The model under review builds one solid part; all positions refer to its coordinate system, in mm. Round coordinates to 2 decimals unless told otherwise and drop trailing zeros. Write each loop counter-clockwise with the first axis right and the second up, starting at its lowest first coordinate (ties: lowest second). Pieces come first, ordered by that corner, then holes.
Item 1: To check wall thickness, follow L1, parallel to Y at x = 187.5, z = 6; L2, parallel to Y at x = 100, z = 3; L3, parallel to Y at x = 35, z = 6.25. State the ranges of each line that lie inside material, in increasing order.
Item 2: Add section D-D (y = 137.3). Give the boundary of the cut face in (x, z).
Item 3: Add section A-A (y = 29). Give the boundary of the cut face in (x, z), plus the area to 3 significant figures.
Item 4: Clearance check with a flat-ended pin moving along its axis: pin 1 Ø4 at (x, z) = (15, 4) entering from -Y. State where the tip first meets the part, or that it passes through.
Item 5: Add section B-B (x = 100). Give the boundary of the cut face in (y, z).
Item 6: Add section C-C (x = 35). Give the boundary of the cut face in (y, z).
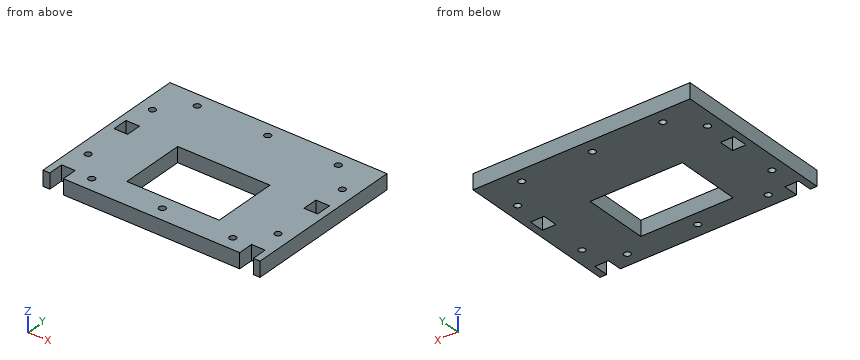
```python
from build123d import *

# Parameters (mm, degrees)
SKETCH1_W                = 200
SKETCH1_H                = 150
BOSS_EXTRUDE1_DEPTH      = 14
SKETCH2_W                = 12.5
SKETCH2_H                = 14
CUT_EXTRUDE1_DEPTH       = 14
F_6_0_6_DIAMETER_HOLE1_D = 6
SKETCH6_W                = 85
SKETCH6_H                = 60
CUT_EXTRUDE2_DEPTH       = 15


with BuildPart() as part:
    # Sketch1 → Boss-Extrude1 (new body)
    with BuildSketch(Plane.XY):
        with Locations((100, 75)):
            Rectangle(SKETCH1_W, SKETCH1_H)
    extrude(amount=BOSS_EXTRUDE1_DEPTH)

    # Sketch2 → Cut-Extrude1 (cut)
    with BuildSketch(Plane(origin=(0, 0, 0), x_dir=(-1, 0, 0), z_dir=(0, 0, -1))):
        with Locations((-12.5, 7)):
            Rectangle(SKETCH2_W, SKETCH2_H)
        with Locations((-187.5, 7)):
            Rectangle(SKETCH2_W, SKETCH2_H)
        with Locations((-12.5, 83)):
            Rectangle(SKETCH2_W, SKETCH2_H)
        with Locations((-187.5, 83)):
            Rectangle(SKETCH2_W, SKETCH2_H)
    extrude(amount=-CUT_EXTRUDE1_DEPTH, mode=Mode.SUBTRACT)

    # Ø6.0 (6) Diameter Hole1 (through all)
    with Locations(Plane.XY.offset(14)):
        with Locations((12.5, 113.265728709), (187.5, 113.265728709), (187.5, 37.265728709), (12.5, 37.265728709), (35, 137.3), (100, 137.3), (165, 137.3), (165, 12.7), (100, 12.7), (35, 12.7)):
            Hole(F_6_0_6_DIAMETER_HOLE1_D / 2)

    # Sketch6 → Cut-Extrude2 (cut, through all)
    with BuildSketch(Plane.XY.offset(14)):
        with Locations((100, 55.4)):
            Rectangle(SKETCH6_W, SKETCH6_H)
    extrude(amount=-CUT_EXTRUDE2_DEPTH, mode=Mode.SUBTRACT)


solid = part.part
```
Numbers:
1. L1: y = 14 to 34.27, 40.27 to 76, 90 to 110.27, 116.27 to 150
1. L2: y = 0 to 9.7, 15.7 to 25.4, 85.4 to 134.3, 140.3 to 150
1. L3: y = 0 to 9.7, 15.7 to 134.3, 140.3 to 150
2. outline: (0, 0) - (32, 0) - (32, 14) - (0, 14) - close; (38, 0) - (97, 0) - (97, 14) - (38, 14) - close; (103, 0) - (162, 0) - (162, 14) - (103, 14) - close; (168, 0) - (200, 0) - (200, 14) - (168, 14) - close
3. outline: (0, 0) - (57.5, 0) - (57.5, 14) - (0, 14) - close; (142.5, 0) - (200, 0) - (200, 14) - (142.5, 14) - close
3. area: 1,610 mm2
4. pin 1: stops at y = 14
5. outline: (0, 0) - (9.7, 0) - (9.7, 14) - (0, 14) - close; (15.7, 0) - (25.4, 0) - (25.4, 14) - (15.7, 14) - close; (85.4, 0) - (134.3, 0) - (134.3, 14) - (85.4, 14) - close; (140.3, 0) - (150, 0) - (150, 14) - (140.3, 14) - close
6. outline: (0, 0) - (9.7, 0) - (9.7, 14) - (0, 14) - close; (15.7, 0) - (134.3, 0) - (134.3, 14) - (15.7, 14) - close; (140.3, 0) - (150, 0) - (150, 14) - (140.3, 14) - close
